Source: CAD feature listing. Evaluate the final solid. Frame: model axes, mm. Face numbers are marked on the shaded views. Coordinates: 2 decimals unless noted, no trailing zeros. Loops run counter-clockwise (first coordinate to the right, second up) from the corner with the lowest first, then second, coordinate; pieces in that order, holes last.
Item 1: Section query A-A, the plane x = -25. Return the cut outline in (y, z), then the cut area to 3 significant figures.
Item 2: Pin query (flat end, axial travel): pin 1 Ø4 at (x, z) = (24.5, 7.5) entering from +Y; pin 2 Ø12 at (x, y) = (5.5, 30.5) entering from +Z; pin 3 Ø4 at (x, z) = (-14.5, 9.5) entering from +Y. Return the tip coordinate at first contact, or that it passes through.
Item 3: Pull-direction query (Y, two-part tool) for the marked faces 1, 2 and 3; classes: +Y half, -Y half, draft (parallel to the pull), parting line (faces both ways), or undercut.
Item 4: Section query B-B, the plane x = 8. Return the cut outline in (y, z), then the cut area to 3 significant figures.
Item 5: Line query: probe 1 along X at (y, z) = (-0.9, 7.5); probe 2 along Y at (x, z) = (-17.5, 0.5); probe 3 along Y at (x, z) = (-18, 0.4). Output: solid intervals per line, ascending.
Item 6: Section query C-C, the plane z = 8. State how many separate pieces and enclosed holes the cut face has, then the cut area to 3 significant figures.
Item 7: Section query D-D, the plane y = 35.5. Return the cut outline in (x, z), then the cut area to 3 significant figures.
```python
from build123d import *

# Parameters (mm, degrees)
SM_BASE_FLANGE_1_DEPTH           = 1.6
SM_EDGE_FLANGE_1_STRIP_W         = 7.8732
SM_EDGE_FLANGE_1_STRIP_H         = 1.6
SM_EDGE_FLANGE_1_STRIP_CUT_DEPTH = 60
SM_EDGE_FLANGE_1_DEPTH           = 60
CUT_EXTRUDE_1_DEPTH              = 56.718578589
SKETCH_9_R                       = 2.1
SKETCH_9_R_2                     = 1.6
SKETCH_9_R_3                     = 4
CUT_EXTRUDE_3_DEPTH              = 10
EXTRUDE_START                    = 1.8
SKETCH_10_R                      = 4.2
SKETCH_10_R_2                    = 2.1
EXTRUDE_2_DEPTH                  = 1.8
SKETCH_11_R                      = 3.2
EXTRUDE_3_DEPTH                  = 1.4
SKETCH_12_R                      = 1.6
CUT_EXTRUDE_4_DEPTH              = 56.398555938


# Sheet-metal steps are written as plain solids
with BuildPart() as part:
    # Sketch 1 → 基体-法兰1 (new body)
    with BuildSketch(Plane.XY):
        Polygon((-26.5, 45), (26.5, 45), (30, 41.5), (30, 0), (-30, 0), (-30, 41.5), align=None)
    extrude(amount=-SM_BASE_FLANGE_1_DEPTH)

    # 边线-法兰1 strip (across the edge) → 边线-法兰1 strip cut (cut)
    with BuildSketch(Plane.YZ.offset(-30)):
        with Locations((-3.2, -0.8)):
            Rectangle(SM_EDGE_FLANGE_1_STRIP_W, SM_EDGE_FLANGE_1_STRIP_H)
    extrude(amount=SM_EDGE_FLANGE_1_STRIP_CUT_DEPTH, mode=Mode.SUBTRACT)

    # 边线-法兰1 section (across the edge) → 边线-法兰1 (add)
    with BuildSketch(Plane.YZ.offset(-30)):
        with BuildLine():
            Line((-1.6, 0.7366), (-1.6, 13.4))
            Line((-1.6, 13.4), (0, 13.4))
            Line((0, 13.4), (0, 0.7366))
            ThreePointArc((0, 0.7366), (0.215745145, 0.215745145), (0.7366, 0))
            Line((0.7366, 0), (0.7366, -1.6))
            ThreePointArc((0.7366, -1.6), (-0.915625705, -0.915625705), (-1.6, 0.7366))
        make_face()
    extrude(amount=SM_EDGE_FLANGE_1_DEPTH)

    # 草图8 → 切除-拉伸1 (cut, through all)
    with BuildSketch(Plane(origin=(0, 0, 0), x_dir=(1, 0, 0), z_dir=(0, 1, 0))):
        Polygon((-30, -11.622497289), (-28.222497289, -13.4), (-30, -13.4), align=None)
        Polygon((28.222497289, -13.4), (30, -13.4), (30, -11.622497289), align=None)
    extrude(amount=-CUT_EXTRUDE_1_DEPTH, mode=Mode.SUBTRACT)

    # 草图9 → 切除-拉伸3 (cut)
    with BuildSketch(Plane(origin=(0, 0, 0), x_dir=(1, 0, 0), z_dir=(0, 1, 0))):
        with Locations(Location((-25, -7.5, 0), (0, 0, 270))):
            Circle(SKETCH_9_R)
        with Locations(Location((-8, -7.5, 0), (0, 0, 270))):
            Circle(SKETCH_9_R_2)
        with Locations(Location((0, -7.5, 0), (0, 0, 270))):
            Circle(SKETCH_9_R_3)
        with Locations(Location((25, -7.5, 0), (0, 0, 270))):
            Circle(SKETCH_9_R)
        with Locations(Location((8, -7.5, 0), (0, 0, 270))):
            Circle(SKETCH_9_R_2)
    extrude(amount=-CUT_EXTRUDE_3_DEPTH, mode=Mode.SUBTRACT)

    # 草图10 → 凸台-拉伸2 (add)
    # profile 1 of 2: a face of its own
    with BuildSketch(Plane(origin=(0, 0, 0), x_dir=(1, 0, 0), z_dir=(0, 1, 0)).offset(EXTRUDE_START)):
        with Locations(Location((-25, -7.5, 0), (0, 0, 270))):
            Circle(SKETCH_10_R)
        with Locations(Location((-25, -7.5, 0), (0, 0, 270))):
            Circle(SKETCH_10_R_2, mode=Mode.SUBTRACT)
    # profile 2 of 2: a face of its own
    with BuildSketch(Plane(origin=(0, 0, 0), x_dir=(1, 0, 0), z_dir=(0, 1, 0)).offset(EXTRUDE_START)):
        with Locations(Location((25, -7.5, 0), (0, 0, 90))):
            Circle(SKETCH_10_R)
        with Locations(Location((25, -7.5, 0), (0, 0, 270))):
            Circle(SKETCH_10_R_2, mode=Mode.SUBTRACT)
    extrude(amount=-EXTRUDE_2_DEPTH)

    # 草图11 → 凸台-拉伸3 (add)
    with BuildSketch(Plane.XY):
        with Locations((-18, 38)):
            Circle(SKETCH_11_R)
        with Locations(Location((18, 38, 0), (0, 0, 180))):
            Circle(SKETCH_11_R)
    extrude(amount=EXTRUDE_3_DEPTH)

    # 草图12 → 切除-拉伸4 (cut, through all)
    with BuildSketch(Plane.XY.offset(1.4)):
        with Locations((-18, 38)):
            Circle(SKETCH_12_R)
        with Locations(Location((18, 38, 0), (0, 0, 180))):
            Circle(SKETCH_12_R)
    extrude(amount=-CUT_EXTRUDE_4_DEPTH, mode=Mode.SUBTRACT)


solid = part.part
```
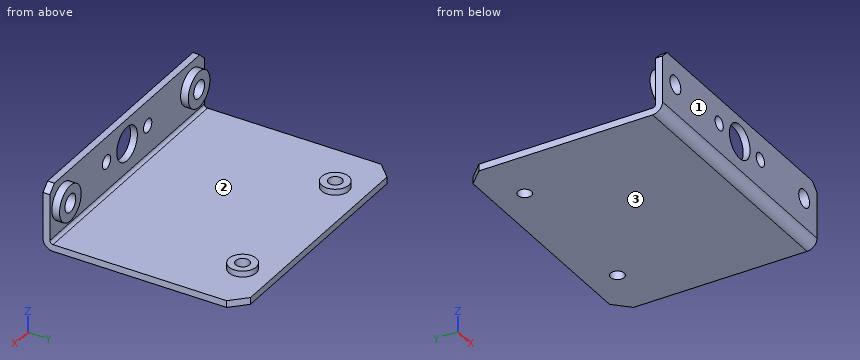
Verdict:
1. outline: (-1.6, 0.74) arc R2.34 ccw to (0.74, -1.6) - (45, -1.6) - (45, 0) - (0.74, 0) arc R0.74 cw to (0, 0.74) - (0, 3.3) - (1.8, 3.3) - (1.8, 5.4) - (-1.6, 5.4) - close; (-1.6, 9.6) - (1.8, 9.6) - (1.8, 11.7) - (0, 11.7) - (0, 13.4) - (-1.6, 13.4) - close
1. area: 95.8 mm2
2. pin 1: stops at y = 1.8
2. pin 2: stops at z = 0
2. pin 3: stops at y = 0
3. face 1: -Y half
3. face 2: undercut
3. face 3: draft
4. outline: (-1.6, 0.74) arc R2.34 ccw to (0.74, -1.6) - (45, -1.6) - (45, 0) - (0.74, 0) arc R0.74 cw to (0, 0.74) - (0, 5.9) - (-1.6, 5.9) - close; (-1.6, 9.1) - (0, 9.1) - (0, 13.4) - (-1.6, 13.4) - close
4. area: 89.8 mm2
5. probe 1: x = -30 to -27.1, -22.9 to -9.6, -6.4 to -4, 4 to 6.4, 9.6 to 22.9, 27.1 to 30
5. probe 2: y = -1.59 to 0.04, 34.84 to 36.48, 39.52 to 41.16
5. probe 3: y = -1.58 to 0.08, 34.8 to 36.4, 39.6 to 41.2
6. separate pieces: 6
6. enclosed holes: 0
6. area: 75.9 mm2
7. outline: (-30, -1.6) - (30, -1.6) - (30, 0) - (20, 0) - (20, 1.4) - (16, 1.4) - (16, 0) - (-16, 0) - (-16, 1.4) - (-20, 1.4) - (-20, 0) - (-30, 0) - close
7. area: 107 mm2
